Check sheet for the drawn part. Datum: minimum x, y, z corner. Units: mm. A direction names the side the tool comes from. Coordinates: 2 decimals unless noted, no trailing zeros. Order: outer loops, then holes, each group sorted by start corner. A loop starts at its lowest first (then second) coordinate and runs counter-clockwise, first axis right, second up.
1. Thickness scan on line 1 (Y direction, x = 6, z = 18.75); line 2 (X direction, y = 10.75, z = 10.5). Record the ranges inside material, lowest first.
2. Cross-section at B-B (z = 14). Enter the section's corners in (x, y).
3. Cross-section at C-C (y = 8.5). Enter the section's corners in (x, z).
4. Draft check along Y on the marked faces 4, 5, 6 and 7. Enter one of: released by +Y, released by -Y, zero draft, split by the parting line, or undercut.
5. Set-up check for the marked faces 1, 2 and 3: record each of +Z, -Z, +X, -X, +Y, -Y from which the full face is reachable in a straight line by a thin tool's end or side.
6. Cross-section at D-D (x = 20.25). Enter the section's corners in (y, z).
7. Gauge pin test, flat ends, axial feed: pin 1 Ø4 at (y, z) = (10.5, 17) entering from +X; pin 2 Ø6.5 at (y, z) = (6.5, 15) entering from -X; pin 3 Ø6 at (x, y) = (16, 10) entering from +Z. Record the tip position at first contact, or that the pin passes through.
8. Cross-section at A-A (x = 7). Enter the section's corners in (y, z).
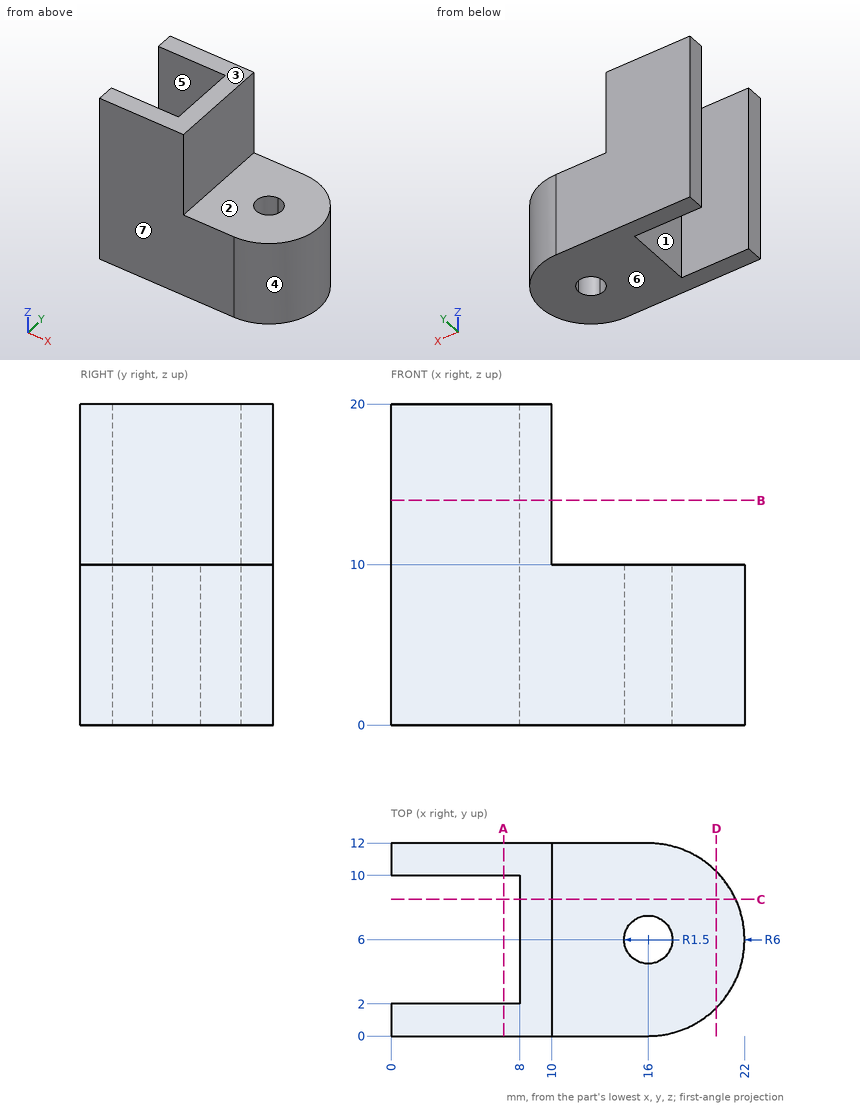
Data:
1. line 1: y = 0 to 2, 10 to 12
1. line 2: x = 0 to 10
2. outline: (0, 0) - (10, 0) - (10, 12) - (0, 12) - (0, 10) - (8, 10) - (8, 2) - (0, 2) - close
3. outline: (8, 0) - (21.45, 0) - (21.45, 10) - (10, 10) - (10, 20) - (8, 20) - close
4. face 4: split by the parting line
4. face 5: undercut
4. face 6: zero draft
4. face 7: released by -Y
5. face 1: +Z, -Z, -X
5. face 2: +Z, +X, +Y, -Y
5. face 3: +Z, +X, -X, +Y, -Y
6. outline: (1.76, 0) - (10.24, 0) - (10.24, 10) - (1.76, 10) - close
7. pin 1: stops at x = 10
7. pin 2: stops at x = 8
7. pin 3: stops at z = 10
8. outline: (0, 0) - (2, 0) - (2, 20) - (0, 20) - close; (10, 0) - (12, 0) - (12, 20) - (10, 20) - close
